Design review of the part shown in the three views and the two pictorial views. Dimensions are in mm from the part's minimum x, y and z. A direction names the side the tool comes from. Coordinates: 2 decimals unless noted, no trailing zeros. Write each loop counter-clockwise with the first axis right and the second up, starting at its lowest first coordinate (ties: lowest second). Pieces come first, ordered by that corner, then holes.
Q1. Take a section at C-C, the plane z = 12. Write out the cut boundary in (x, y).
Q2. For L1, parallel to Y at x = 6.5, z = 42.5, list the stretches that pass through material, from the lowest coordinate up.
Q3. For the marked faces 1 and 2, list the 3-axis set-ups (+Z, -Z, +X, -X, +Y, -Y) from which the entire face can be reached by the end or side of a thin tool; tool diameter is ignored.
Q4. Take a section at A-A, the plane z = 25. Write out the cut boundary in (x, y), plus the area to 3 significant figures.
Q5. For pin 1 Ø1.5 at (x, y) = (31.5, 9.5) entering from -Z; pin 2 Ø1 at (x, z) = (21.5, 31) entering from -Y, all flat-tipped, find the tip position at first contact; note any pin that passes through.
Q6. Take a section at D-D, the plane x = 41. Write out the cut boundary in (y, z), plus the area to 3 significant figures.
Q7. Take a section at B-B, the plane x = 25. Write out the cut boundary in (y, z), plus the area to 3 significant figures.
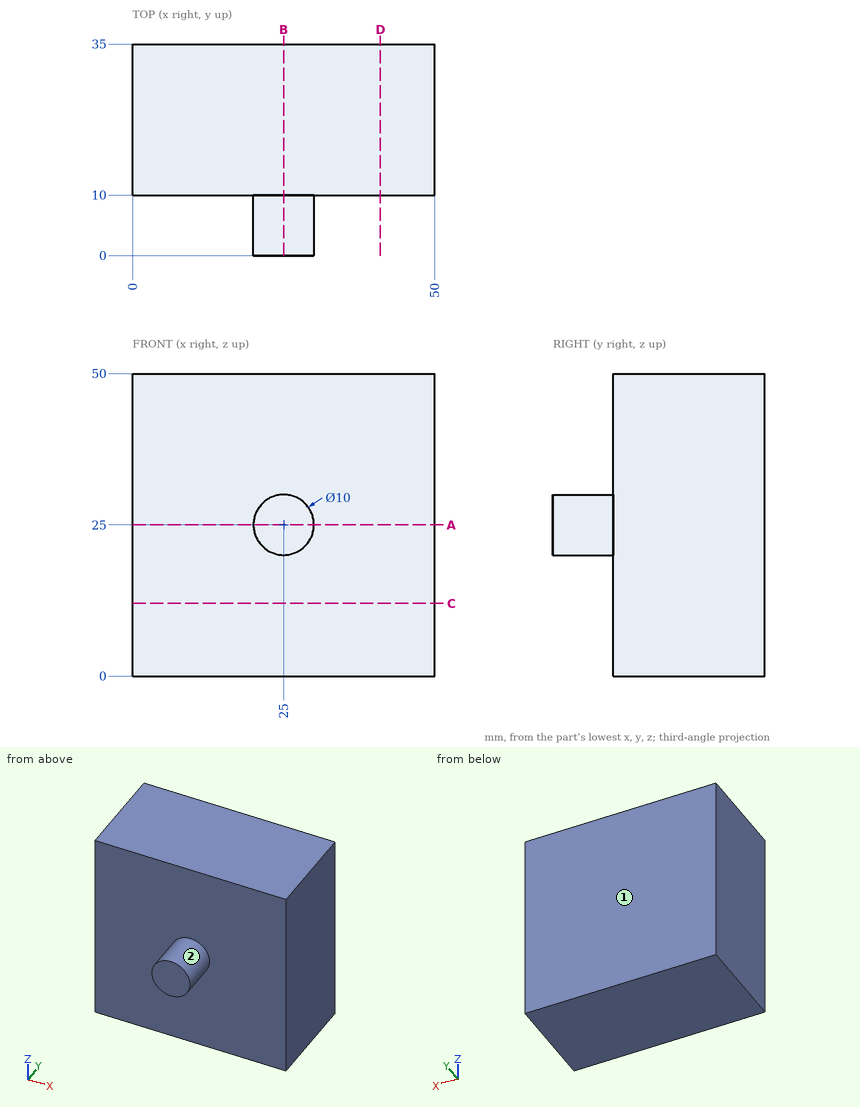
Responses:
1. outline: (0, 10) - (50, 10) - (50, 35) - (0, 35) - close
2. L1: y = 10 to 35
3. face 1: +Z, -Z, +X, -X, +Y
3. face 2: -Y
4. outline: (0, 10) - (20, 10) - (20, 0) - (30, 0) - (30, 10) - (50, 10) - (50, 35) - (0, 35) - close
4. area: 1,350 mm2
5. pin 1: stops at z = 0
5. pin 2: stops at y = 10
6. outline: (10, 0) - (35, 0) - (35, 50) - (10, 50) - close
6. area: 1,250 mm2
7. outline: (0, 20) - (10, 20) - (10, 0) - (35, 0) - (35, 50) - (10, 50) - (10, 30) - (0, 30) - close
7. area: 1,350 mm2
